```python
from build123d import *

# Parameters (mm, degrees)
BOSS_EXTRUDE1_DEPTH       = 8
CUT_EXTRUDE1_DEPTH        = 8
SKETCH7_R                 = 1.5
CUT_EXTRUDE4_DEPTH        = 6
SKETCH9_R                 = 2.5
CUT_EXTRUDE5_DEPTH        = 15
CUT_EXTRUDE2_DEPTH        = 21
CUT_EXTRUDE3_DEPTH        = 21
M2X0_4_TAPPED_HOLE1_D     = 1.6
M2X0_4_TAPPED_HOLE1_DEPTH = 8
M2X0_4_TAPPED_HOLE1_TIP   = 0.480688495
FILLET1_R                 = 1
FILLET2_R                 = 1


with BuildPart() as part:
    # Sketch1 → Boss-Extrude1 (new body)
    with BuildSketch(Plane.XY):
        Polygon((0, 0), (0, 42), (20, 42), (20, 20), (40, 20), (40, 12), align=None)
    extrude(amount=BOSS_EXTRUDE1_DEPTH)

    # Sketch2 → Cut-Extrude1 (cut)
    with BuildSketch(Plane.XY.offset(8)):
        Polygon((15, 42), (15, 35), (0, 28), (0, 42), align=None)
    extrude(amount=-CUT_EXTRUDE1_DEPTH, mode=Mode.SUBTRACT)

    # Sketch7 → Cut-Extrude4 (cut)
    with BuildSketch(Plane(origin=(0, 20, 0), x_dir=(1, 0, 0), z_dir=(0, 1, 0))):
        with Locations((34, -4)):
            Circle(SKETCH7_R)
        with Locations((26, -4)):
            Circle(SKETCH7_R)
    extrude(amount=-CUT_EXTRUDE4_DEPTH, mode=Mode.SUBTRACT)

    # Sketch9 → Cut-Extrude5 (cut, through all)
    with BuildSketch(Plane(origin=(0, 14, 0), x_dir=(1, 0, 0), z_dir=(0, 1, 0))):
        with Locations((34, -4)):
            Circle(SKETCH9_R)
        with Locations((26, -4)):
            Circle(SKETCH9_R)
    extrude(amount=-CUT_EXTRUDE5_DEPTH, mode=Mode.SUBTRACT)

    # Sketch5 → Cut-Extrude2 (cut, through all)
    with BuildSketch(Plane(origin=(20, 0, 0), x_dir=(0, 0, -1), z_dir=(1, 0, 0))):
        Polygon((-8, 42), (-4, 42), (-8, 38), align=None)
    extrude(amount=-CUT_EXTRUDE2_DEPTH, mode=Mode.SUBTRACT)

    # Sketch6 → Cut-Extrude3 (cut, through all)
    with BuildSketch(Plane(origin=(20, 0, 0), x_dir=(0, 0, -1), z_dir=(1, 0, 0))):
        Polygon((0, 42), (-4, 42), (0, 38), align=None)
    extrude(amount=-CUT_EXTRUDE3_DEPTH, mode=Mode.SUBTRACT)

    # M2x0.4 Tapped Hole1
    with Locations(Plane(origin=(0, 24, 4), x_dir=(0, 0, -1), z_dir=(-1, 0, 0))):
        with Locations((0, 0), (0, 8), (0, 16)):
            Hole(M2X0_4_TAPPED_HOLE1_D / 2, depth=M2X0_4_TAPPED_HOLE1_DEPTH)
            with Locations((0, 0, -(M2X0_4_TAPPED_HOLE1_DEPTH + M2X0_4_TAPPED_HOLE1_TIP / 2))):  # 118° drill point
                Cone(0, M2X0_4_TAPPED_HOLE1_D / 2, M2X0_4_TAPPED_HOLE1_TIP, mode=Mode.SUBTRACT)

    # Fillet1
    fillet1_edges = [part.edges().sort_by_distance(p)[0] for p in [
        (20, 20, 4),
    ]]
    fillet(fillet1_edges, radius=FILLET1_R)

    # Fillet2
    fillet2_edges = [part.edges().sort_by_distance(p)[0] for p in [
        (15, 35, 4),
    ]]
    fillet(fillet2_edges, radius=FILLET2_R)


solid = part.part
```
Work out the finished part from the listing and answer in its coordinate system (mm). A direction names the side the tool comes from. Round coordinates to 2 decimals unless told otherwise and drop trailing zeros. Loops run counter-clockwise (first coordinate to the right, second up) from the corner with the lowest first, then second, coordinate; pieces in that order, holes last.
(1) The part is cut by section B-B, the plane z = 7.5. Give the vertices of the cut face in (x, y), and give its area (3 significant figures).
Computed values:
outline: (0, 0) - (40, 12) - (40, 20) - (21, 20) arc R1 cw to (20, 21) - (20, 38.5) - (15, 38.5) - (15, 35.64) arc R1 cw to (14.42, 34.73) - (0, 28) - close
area: 825 mm2
(2) Find the intervals of material crossed by L1, parallel to X at y = 16.1, z = 4; L2, parallel to Z at x = 3.25, y = 24; L3, parallel to Z at x = 26, y = 10, in increasing order.
Computed values:
L1: x = 8.42 to 24.5, 27.5 to 32.5, 35.5 to 40
L2: z = 0 to 3.2, 4.8 to 8
L3: z = 0 to 1.5, 6.5 to 8
(3) The part is cut by section C-C, the plane x = 19.5. Give the vertices of the cut face in (y, z), and give its area (3 significant figures).
Computed values:
outline: (5.85, 0) - (38, 0) - (42, 4) - (38, 8) - (5.85, 8) - close
area: 273 mm2
(4) The mould has two halves that part along Z. Classify faces 6 (the flat face through (18, 40, 2)), 7 (the cylindrical face through (31.5, 12.2, 3.9)), 8 (the flat face through (20, 32, 4)): pulls with the +Z half, pulls with the -Z half, needs draft (parallel to the pull), parting line crosses it, or undercut.
Computed values:
face 6: pulls with the -Z half
face 7: undercut
face 8: needs draft
(5) The part is cut by section D-D, the plane y = 34. Give the vertices of the cut face in (x, z).
Computed values:
outline: (12.86, 0) - (20, 0) - (20, 8) - (12.86, 8) - close
(6) Each of these flat-tipped pins is pushed along its axis until it touches: P1, Ø1.5, axis at y = 24, z = 2.5, coming from the +X side; P2, Ø2, axis at x = 8, z = 6.5, coming from the +Y side; P3, Ø2.5, axis at x = 30, z = 4, coming from the +Y side; P4, Ø1.5, axis at x = 26, z = 3.5, coming from the -Y side. Where does it stop, or does it pass through?
Computed values:
P1: stops at x = 20
P2: stops at y = 32.2
P3: stops at y = 20
P4: passes through
(7) For faces 1 (the cylindrical face through (23.5, 10.5, 3.9)), 2 (the flat face through (30, 20, 4)), 3 (the cylindrical face through (4.06, 7.46, 3.41)), 4 (the flat face through (15, 38, 4)), 5 (the cylindrical face through (24.5, 17.04, 3.93)), determine the directions among +Z, -Z, +X, -X, +Y, -Y from which every point of the face is accessible in a straight line to the end or side of a thin tool.
Computed values:
face 1: -Y
face 2: +Z, -Z, +X, +Y
face 3: -X
face 4: +Z, -Z, -X, +Y
face 5: +Y, -Y
(8) The part is cut by section A-A, the plane x = 34. Give the vertices of the cut face in (y, z), and give its area (3 significant figures).
Computed values:
outline: (10.2, 0) - (20, 0) - (20, 2.5) - (14, 2.5) - (14, 1.5) - (10.2, 1.5) - close; (10.2, 6.5) - (14, 6.5) - (14, 5.5) - (20, 5.5) - (20, 8) - (10.2, 8) - close
area: 41.4 mm2
